Can you work these out from the model? Positions are in its coordinate system, mm. Face numbers are marked on the shaded views. Round coordinates to 2 decimals unless told otherwise and drop trailing zeros. Loops run counter-clockwise (first coordinate to the right, second up) from the corner with the lowest first, then second, coordinate; pieces in that order, holes last. Notation, with made-up numbers: (-12.5, 75) -> (-7.5, 75) arc R14 ccw to (-7.5, 98) -> close; hole circle Ø5 at (82, 53.5). An arc over 180 degrees is marked (long way). Use a Markdown table: item, result.
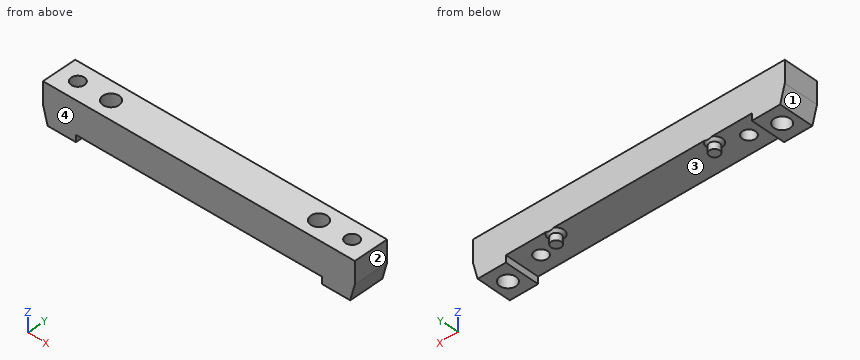
from build123d import *
from OCP.BRepFilletAPI import BRepFilletAPI_MakeChamfer

# Parameters (mm, degrees)
SKETCH2_W                       = 90
SKETCH2_H                       = 10
BOSS_EXTRUDE1_DEPTH             = 9.35
SKETCH4_W                       = 9.5
SKETCH4_H                       = 10
BOSS_EXTRUDE2_DEPTH             = 2
SKETCH5_R                       = 1.45
BOSS_EXTRUDE3_DEPTH             = 2.8
CHAMFER1_SIZE                   = 0.8
CHAMFER2_SIZE                   = 5
CHAMFER2_SIZE2                  = 1.339745962
F_13_0_185_DIAMETER_HOLE1_D     = 4.699
F_13_0_185_DIAMETER_HOLE1_DEPTH = 6.35
F_6_CLEARANCE_HOLE1_D           = 3.7973
F_6_CLEARANCE_HOLE1_ON_FACE_2_D = 3.7973
F_13_0_185_DIAMETER_HOLE2_D     = 4.699
F_13_0_185_DIAMETER_HOLE2_DEPTH = 6.35
F_6_CLEARANCE_HOLE2_D           = 3.7973


with BuildPart() as part:
    # Sketch2 → Boss-Extrude1 (new body)
    with BuildSketch(Plane.XY):
        with Locations((45, 5)):
            Rectangle(SKETCH2_W, SKETCH2_H)
    extrude(amount=BOSS_EXTRUDE1_DEPTH)

    # Sketch4 → Boss-Extrude2 (add)
    with BuildSketch(Plane(origin=(0, 0, 0), x_dir=(-1, 0, 0), z_dir=(0, 0, -1))):
        with Locations((-4.75, 5)):
            Rectangle(SKETCH4_W, SKETCH4_H)
        with Locations((-85.25, 5)):
            Rectangle(SKETCH4_W, SKETCH4_H)
    extrude(amount=BOSS_EXTRUDE2_DEPTH)

    # Sketch5 → Boss-Extrude3 (add)
    with BuildSketch(Plane(origin=(0, 0, 0), x_dir=(-1, 0, 0), z_dir=(0, 0, -1))):
        with Locations(Location((-67.863406388, 8.0148451, 0), (0, 0, 180))):
            Circle(SKETCH5_R)
        with Locations(Location((-22.143406388, 8.0148451, 0), (0, 0, 180))):
            Circle(SKETCH5_R)
    extrude(amount=BOSS_EXTRUDE3_DEPTH)

    # Chamfer1
    # the kernel refuses this chamfer: 0.8 mm, written as the material it adds along each edge
    with BuildSketch(Plane(origin=(67.863406388, 8.0148451, 0), x_dir=(1, 0, 0), z_dir=(0, 1, 0))) as chamfer1_piece_1_section:
        Polygon((1.45 + CHAMFER1_SIZE, 0), (1.45, CHAMFER1_SIZE), (1.45, 0), align=None)
    chamfer1_piece_1 = revolve(axis=Axis((67.863406388, 8.0148451, 0), (0, 0, -1)), mode=Mode.PRIVATE)
    chamfer1_piece_1 = split(chamfer1_piece_1, bisect_by=Plane(origin=(66.024382204, 10, -0.389024184), z_dir=(0, -1, 0)), keep=Keep.TOP, mode=Mode.PRIVATE)
    add(chamfer1_piece_1)
    with BuildSketch(Plane(origin=(22.143406388, 8.0148451, 0), x_dir=(1, 0, 0), z_dir=(0, 1, 0))) as chamfer1_piece_2_section:
        Polygon((1.45 + CHAMFER1_SIZE, 0), (1.45, CHAMFER1_SIZE), (1.45, 0), align=None)
    chamfer1_piece_2 = revolve(axis=Axis((22.143406388, 8.0148451, 0), (0, 0, -1)), mode=Mode.PRIVATE)
    chamfer1_piece_2 = split(chamfer1_piece_2, bisect_by=Plane(origin=(20.304382204, 10, -0.389024184), z_dir=(0, -1, 0)), keep=Keep.TOP, mode=Mode.PRIVATE)
    add(chamfer1_piece_2)

    # Chamfer2: one chamfer whose edges measure the first distance from different faces: ONE call of the kernel's chamfer builder (chamfer() names one face for all edges)
    chamfer2_edges_1 = [part.edges().sort_by_distance(p)[0] for p in [
        (0, 5, -2),
    ]]
    chamfer2_side_1 = [part.faces().sort_by_distance(p)[0] for p in [
        (0, 5, 3.675),
    ]]
    chamfer2_edges_2 = [part.edges().sort_by_distance(p)[0] for p in [
        (90, 5, -2),
    ]]
    chamfer2_side_2 = [part.faces().sort_by_distance(p)[0] for p in [
        (90, 5, 3.675),
    ]]
    chamfer2 = BRepFilletAPI_MakeChamfer(part.part.solid().wrapped)
    for e in chamfer2_edges_1:
        chamfer2.Add(CHAMFER2_SIZE, CHAMFER2_SIZE2, e.wrapped, chamfer2_side_1[0].wrapped)  # the first distance lies on this face
    for e in chamfer2_edges_2:
        chamfer2.Add(CHAMFER2_SIZE, CHAMFER2_SIZE2, e.wrapped, chamfer2_side_2[0].wrapped)  # the first distance lies on this face
    add(Compound.cast(chamfer2.Shape()), mode=Mode.REPLACE)

    # #13 (0.185) Diameter Hole1
    with Locations(Plane(origin=(84.580127019, 5, -2), x_dir=(-1, 0, 0), z_dir=(0, 0, -1))):
        with Locations((0, 0), (79.160254038, 0)):
            Hole(F_13_0_185_DIAMETER_HOLE1_D / 2, depth=F_13_0_185_DIAMETER_HOLE1_DEPTH)

    # #6 Clearance Hole1 (through all)
    with Locations(Plane(origin=(84.580127019, 5, 4.35), x_dir=(-1, 0, 0), z_dir=(0, 0, -1))):
        with Locations((0, 0), (79.160254038, 0)):
            Hole(F_6_CLEARANCE_HOLE1_D / 2)

    # #6 Clearance Hole1 on face 2 (through all)
    with Locations(Plane(origin=(5.419872981, 5, 0), x_dir=(-1, 0, 0), z_dir=(0, 0, -1))):
        with Locations((0, 0)):
            Hole(F_6_CLEARANCE_HOLE1_ON_FACE_2_D / 2)

    # #13 (0.185) Diameter Hole2
    with Locations(Plane(origin=(75, 5, 9.35), x_dir=(1, 0, 0), z_dir=(0, 0, 1))):
        with Locations((0, 0), (-60, 0)):
            Hole(F_13_0_185_DIAMETER_HOLE2_D / 2, depth=F_13_0_185_DIAMETER_HOLE2_DEPTH)

    # #6 Clearance Hole2 (through all)
    with Locations(Plane(origin=(75, 5, 3), x_dir=(1, 0, 0), z_dir=(0, 0, 1))):
        with Locations((0, 0), (-60, 0)):
            Hole(F_6_CLEARANCE_HOLE2_D / 2)


solid = part.part
1. I want a section at D-D (x = 33.5). Please give me the cut outline in (y, z).
Answer sheet:
| item | result |
|---|---|
| outline | (0, 0) -> (10, 0) -> (10, 9.35) -> (0, 9.35) -> close |
2. I want a section at B-B (y = 1). Please give me the cut outline in (x, z).
Answer sheet:
| item | result |
|---|---|
| outline | (0, 3) -> (1.34, -2) -> (9.5, -2) -> (9.5, 0) -> (80.5, 0) -> (80.5, -2) -> (88.66, -2) -> (90, 3) -> (90, 9.35) -> (0, 9.35) -> close |
3. Will these pins go through, and if not, where does the flat tip stop? pin 1 Ø4 at (x, y) = (15, 5) entering from -Z; pin 2 Ø0.6 at (y, z) = (7, -1) entering from -X; pin 3 Ø2.5 at (x, y) = (4.5, 4.5) entering from -Z.
Answer sheet:
| item | result |
|---|---|
| pin 1 | stops at z = 0 |
| pin 2 | stops at x = 0.99 |
| pin 3 | stops at z = 4.35 |
4. I want a section at C-C (y = 5). State how many separate pieces and enclosed holes the cut face has, plus the area to 3 significant figures.
Answer sheet:
| item | result |
|---|---|
| separate pieces | 5 |
| enclosed holes | 0 |
| area | 693 mm² |
5. If we mould it in two halves opening along X, with no side actions, what happens to the marked faces 1, 2, 3 and 4? For each: +X half, -X half, draft (parallel to the pull), parting line (faces both ways), or undercut.
Answer sheet:
| item | result |
|---|---|
| face 1 | -X half |
| face 2 | +X half |
| face 3 | undercut |
| face 4 | draft |
6. I want a section at A-A (x = 15). Please give me the cut outline in (y, z), plus the area to 3 significant figures.
Answer sheet:
| item | result |
|---|---|
| outline | (0, 0) -> (3.1, 0) -> (3.1, 3) -> (2.65, 3) -> (2.65, 9.35) -> (0, 9.35) -> close; (6.9, 0) -> (10, 0) -> (10, 9.35) -> (7.35, 9.35) -> (7.35, 3) -> (6.9, 3) -> close |
| area | 52.3 mm² |
7. I need wall thicknesses on line 1 (X direction, y = 5.5, z = 8.75); line 2 (X direction, y = 4.75, z = 2); line 3 (X direction, y = 5.5, z = -0.5). Which ranges of each line are inside material? Lowest first, please.
Answer sheet:
| item | result |
|---|---|
| line 1 | x = 0 to 3.59, 7.25 to 12.7, 17.3 to 72.7, 77.3 to 82.75, 86.41 to 90 |
| line 2 | x = 0.27 to 3.08, 7.76 to 13.12, 16.88 to 73.12, 76.88 to 82.24, 86.92 to 89.73 |
| line 3 | x = 0.94 to 3.12, 7.72 to 9.5, 80.5 to 82.28, 86.88 to 89.06 |
